Verification items for the finished model (mm, model axes). A direction names the side the tool comes from. Round coordinates to 2 decimals unless told otherwise and drop trailing zeros. Write each loop counter-clockwise with the first axis right and the second up, starting at its lowest first coordinate (ties: lowest second). Pieces come first, ordered by that corner, then holes. Notation, with made-up numbers: (71.5, 30.5) -> (128.5, 30.5) arc R8 cw to (128.5, 45.5) -> close; hole circle Ø2 at (-35, 8.5). An arc over 180 degrees is marked (long way). Answer as a JSON object with one key per item and string values. Group by question number.
(1) Scan lines: L1, parallel to Z at x = -26, y = 27.5; L2, parallel to X at y = 4, z = 16.5; L3, parallel to X at y = 21, z = 0. Record each from-to range of solid material in increasing order. Write a range as from..to.
(2) Gauge pin test, flat ends, axial feed: pin 1 Ø7.5 at (y, z) = (32.5, 19.5) entering from -X; pin 2 Ø13 at (x, z) = (-53, 13) entering from -Y; pin 3 Ø4 at (x, y) = (48, 5) entering from -Z; pin 4 Ø1.5 at (y, z) = (37, -8) entering from -X. Record the tip position at first contact, or that the pin passes through.
(3) Draft check along Y on faces 5 (the face through (4.82, 36.64, -19.55)), 6 (the face through (-30, 8, 0)), 7 (the face through (-37.9, 50.4, 0.3)), 8 (the face through (-21, 23, -23)). Enter one of: released by +Y, released by -Y, zero draft, split by the parting line, or undercut.
(4) Sectioned sample at A-A on z = 0. Record the cut outline in (x, y).
(5) Sectioned sample at D-D on y = 11. Record the cut outline in (x, z), and give its area (3 significant figures).
(6) Sectioned sample at B-B on x = -32. Record the cut outline in (y, z).
(7) Sectioned sample at C-C on x = -53. Record the cut outline in (y, z).
(8) Set-up check for faces 1 (the face through (11.241, 23.997, -5.076)), 2 (the face through (-16, 27, -16)), 3 (the face through (-46, 27, -20)), 4 (the face through (16, 28, -5)): record each of +Z, -Z, +X, -X, +Y, -Y from which the full face is reachable in a straight line by a thin tool's end or side.
```python
from build123d import *

# Parameters (mm, degrees)
SKETCH1_R                = 4
BOSS_EXTRUDE1_DEPTH      = 8
BOSS_EXTRUDE2_DEPTH      = 5
BOSS_EXTRUDE2_DEPTH_BACK = 51
BOSS_EXTRUDE3_DEPTH      = 7
BOSS_EXTRUDE5_REACH      = 46
SKETCH7_R                = 14
SKETCH4_R                = 11
BOSS_EXTRUDE4_DEPTH      = 28
CUT_EXTRUDE1_REACH       = 58
SKETCH5_R                = 14
SKETCH5_R_2              = 8
SKETCH6_R                = 6
CUT_EXTRUDE2_DEPTH       = 28


with BuildPart() as part:
    # Sketch1 → Boss-Extrude1 (new body)
    with BuildSketch(Plane(origin=(0, 0, 0), x_dir=(1, 0, 0), z_dir=(0, 1, 0))):
        with BuildLine():
            Line((55, -23), (-55, -23))
            ThreePointArc((-55, -23), (-60.656854249, -20.656854249), (-63, -15))
            Line((-63, -15), (-63, 15))
            ThreePointArc((-63, 15), (-60.656854249, 20.656854249), (-55, 23))
            Line((-55, 23), (55, 23))
            ThreePointArc((55, 23), (60.656854249, 20.656854249), (63, 15))
            Line((63, 15), (63, -15))
            ThreePointArc((63, -15), (60.656854249, -20.656854249), (55, -23))
        make_face()
        with Locations(Location((-53, 13, 0), (0, 0, 270))):  # turned: the seam where the file's is
            Circle(SKETCH1_R, mode=Mode.SUBTRACT)
        with Locations(Location((53, 13, 0), (0, 0, 270))):  # turned: the seam where the file's is
            Circle(SKETCH1_R, mode=Mode.SUBTRACT)
        with Locations(Location((-53, -13, 0), (0, 0, 270))):  # turned: the seam where the file's is
            Circle(SKETCH1_R, mode=Mode.SUBTRACT)
        with Locations(Location((53, -13, 0), (0, 0, 270))):  # turned: the seam where the file's is
            Circle(SKETCH1_R, mode=Mode.SUBTRACT)
    extrude(amount=BOSS_EXTRUDE1_DEPTH)

    # Sketch2 → Boss-Extrude2 (add, two sides)
    with BuildSketch(Plane.XY.offset(23)) as boss_extrude2_sk:
        with BuildLine():
            Line((0, 0), (42, 0))
            ThreePointArc((42, 0), (21, 21), (0, 0))
        make_face()
    extrude(amount=BOSS_EXTRUDE2_DEPTH)
    extrude(boss_extrude2_sk.sketch, amount=-BOSS_EXTRUDE2_DEPTH_BACK)

    # Sketch3 → Boss-Extrude3 (add)
    with BuildSketch(Plane.XY.offset(23)):
        with BuildLine():
            Line((-46, 45), (-46, 0))
            Line((-46, 0), (0, 0))
            ThreePointArc((0, 0), (11.23098253, 18.589413591), (32.911075968, 17.295267251))
            Line((32.911075968, 17.295267251), (-24.059282688, 56.530178167))
            ThreePointArc((-24.059282688, 56.530178167), (-38.512678314, 57.392942394), (-46, 45))
        make_face()
    boss_extrude3 = extrude(amount=-BOSS_EXTRUDE3_DEPTH)

    # Mirror1: Boss-Extrude3 across plane
    add(boss_extrude3.mirror(Plane.XY))

    # Sketch7 → Boss-Extrude5 (add, up to next)
    with BuildSketch(Plane(origin=(0, 0, 16), x_dir=(-1, 0, 0), z_dir=(0, 0, -1)), mode=Mode.PRIVATE) as boss_extrude5_sk1:
        with Locations(Location((32, 45, 0), (0, 0, 124.554792234))):  # turned: the seam where the file's is
            Circle(SKETCH7_R)
    boss_extrude5_tool1 = extrude(boss_extrude5_sk1.sketch, amount=BOSS_EXTRUDE5_REACH, mode=Mode.PRIVATE) - part.part
    add(boss_extrude5_tool1.solids().sort_by_distance((-32, 45, 16))[0])

    # Sketch4 → Boss-Extrude4 (add)
    with BuildSketch(Plane.XZ):
        with Locations(Location((21, 0, 0), (0, 0, 270))):  # turned: the seam where the file's is
            Circle(SKETCH4_R)
    extrude(amount=-BOSS_EXTRUDE4_DEPTH)

    # Sketch5 → Cut-Extrude1 (cut, up to next)
    with BuildSketch(Plane.XY.offset(28), mode=Mode.PRIVATE) as cut_extrude1_sk1:
        with Locations((21, 0)):
            Circle(SKETCH5_R)
    cut_extrude1_tool1 = extrude(cut_extrude1_sk1.sketch, amount=-CUT_EXTRUDE1_REACH, mode=Mode.PRIVATE) & part.part
    add(cut_extrude1_tool1.solids().sort_by_distance((21, 0, 28))[0], mode=Mode.SUBTRACT)
    # Sketch5 → Cut-Extrude1 (cut, up to next)
    with BuildSketch(Plane.XY.offset(28), mode=Mode.PRIVATE) as cut_extrude1_sk2:
        with Locations((-32, 45)):
            Circle(SKETCH5_R_2)
    cut_extrude1_tool2 = extrude(cut_extrude1_sk2.sketch, amount=-CUT_EXTRUDE1_REACH, mode=Mode.PRIVATE) & part.part
    add(cut_extrude1_tool2.solids().sort_by_distance((-32, 45, 28))[0], mode=Mode.SUBTRACT)

    # Sketch6 → Cut-Extrude2 (cut)
    with BuildSketch(Plane(origin=(0, 28, 0), x_dir=(1, 0, 0), z_dir=(0, 1, 0))):
        with Locations(Location((21, 0, 0), (0, 0, 270))):  # turned: the seam where the file's is
            Circle(SKETCH6_R)
    extrude(amount=-CUT_EXTRUDE2_DEPTH, mode=Mode.SUBTRACT)


solid = part.part
```
Computed values:
{
 "1": {"L1": "-23..-16, 16..23", "L2": "-62.86..-54.94, -51.06..7.58, 34.42..51.06, 54.94..62.86", "L3": "10..15, 27..32"},
 "2": {"pin 1": "x = -46", "pin 2": "y = 0", "pin 3": "z = -23", "pin 4": "x = -43.98"},
 "3": {"face 5": "released by +Y", "face 6": "undercut", "face 7": "undercut", "face 8": "zero draft"},
 "4": {"outline": "(-63, 0) -> (7, 0) arc R14 cw to (15, 12.65) -> (15, 28) -> (10, 28) -> (10, 17.89) arc R21 ccw to (1.58, 8) -> (-63, 8) -> close; circle Ø28 at (-32, 45); (27, 12.65) arc R14 cw to (35, 0) -> (63, 0) -> (63, 8) -> (40.42, 8) arc R21 ccw to (32, 17.89) -> (32, 28) -> (27, 28) -> close; hole circle Ø16 at (-32, 45)"},
 "5": {"outline": "(-46, -23) -> (3.11, -23) -> (3.11, -28) -> (12.34, -28) -> (12.34, 28) -> (3.11, 28) -> (3.11, 23) -> (-46, 23) -> (-46, 16) -> (3.11, 16) -> (3.11, -16) -> (-46, -16) -> close; (29.66, -28) -> (38.89, -28) -> (38.89, 28) -> (29.66, 28) -> close", "area": "1,720 mm2"},
 "6": {"outline": "(0, -23) -> (37, -23) -> (37, 23) -> (0, 23) -> close; (53, -23) -> (59, -23) -> (59, 23) -> (53, 23) -> close; hole (8, -16) -> (31, -16) -> (31, 16) -> (8, 16) -> close"},
 "7": {"outline": "(0, -23) -> (8, -23) -> (8, -17) -> (0, -17) -> close; (0, -9) -> (8, -9) -> (8, 9) -> (0, 9) -> close; (0, 17) -> (8, 17) -> (8, 23) -> (0, 23) -> close"},
 "8": {"face 1": "+Y", "face 2": "none", "face 3": "+Z, -Z, -X, +Y", "face 4": "+X, -X, +Y"}
}
